For this review, take the finished solid that the model builds, in its own axes (mm). A direction names the side the tool comes from. Give positions to 0.01 mm unless a question says otherwise; leave off trailing zeros. Write each loop counter-clockwise with the first axis right and the second up, starting at its lowest first coordinate (ties: lowest second). Pieces come first, ordered by that corner, then holes. Notation, with made-up numbers: (-30, 22.5) -> (-4, 22.5) arc R22 ccw to (-4, 29.5) -> close; hole circle Ø11 at (83, 27). An arc over 180 degrees is marked (long way). Return JSON: item names as keys, results as strings.
from build123d import *

# Parameters (mm, degrees)
SKETCH1_W           = 139.457769838
SKETCH1_H           = 99.02864438
BOSS_EXTRUDE1_DEPTH = 10
BOSS_EXTRUDE2_DEPTH = 99.028644381
BOSS_EXTRUDE3_DEPTH = 99.028644381


with BuildPart() as part:
    # Sketch1 → Boss-Extrude1 (new body)
    with BuildSketch(Plane.XY):
        Rectangle(SKETCH1_W, SKETCH1_H)
    extrude(amount=BOSS_EXTRUDE1_DEPTH)

    # Sketch2 → Boss-Extrude2 (add)
    with BuildSketch(Plane(origin=(0, 49.51432219, 0), x_dir=(1, 0, 0), z_dir=(0, 1, 0))):
        Polygon((-69.728884919, 0), (41.491223437, 119.146703645), (25.829944634, 119.146703645), (-103.609221326, -10), (-69.728884919, -10), align=None)
    extrude(amount=-BOSS_EXTRUDE2_DEPTH)

    # Sketch3 → Boss-Extrude3 (add)
    with BuildSketch(Plane(origin=(0, 49.51432219, 0), x_dir=(1, 0, 0), z_dir=(0, 1, 0))):
        Polygon((41.491223437, 119.146703645), (41.491223437, 283.914864742), (-131.976237247, 283.914864742), (-131.976237247, 227.19452677), (25.829944634, 227.19452677), (25.829944634, 119.146703645), align=None)
    extrude(amount=-BOSS_EXTRUDE3_DEPTH)


solid = part.part
1. For pin 1 (2 mm diameter, centred on y = -25.5, z = -106, fed in from +X); pin 2 (8 mm diameter, centred on y = -5.5, z = -254.5, fed in from +X), all flat-tipped, find the tip position at first contact; note any pin that passes through.
Results found:
{"pin 1": "stops at x = 30.15", "pin 2": "stops at x = 41.49"}
2. The part is to be moulded in two halves that separate along Z. For faces 1 (the flat face through (25.83, 1, -174)), 2 (the flat face through (-44, 1, -283.915)), 3 (the flat face through (-47, 49.514, -236)), 4 (the flat face through (-1, 1, 0)), say which applies: +Z half, -Z half, draft (parallel to the pull), parting line (faces both ways), or undercut.
Results found:
{"face 1": "undercut", "face 2": "-Z half", "face 3": "draft", "face 4": "undercut"}
3. For faces 5 (the flat face through (-37.98, 0.69, -55.48)), 6 (the flat face through (41.491, 1, -200)), 7 (the flat face through (-14.897, 0.693, -58.739)), 8 (the flat face through (69.729, -1, 5)), list the 3-axis set-ups (+Z, -Z, +X, -X, +Y, -Y) from which the entire face can be reached by the end or side of a thin tool; tool diameter is ignored.
Results found:
{"face 5": "-X, +Y, -Y", "face 6": "-Z, +X, +Y, -Y", "face 7": "+X, +Y, -Y", "face 8": "+Z, -Z, +X, +Y, -Y"}
4. Add section B-B, the plane y = -17. State the section outline as (x, z) points.
Results found:
{"outline": "(-131.98, -283.91) -> (41.49, -283.91) -> (41.49, -119.15) -> (-69.73, 0) -> (69.73, 0) -> (69.73, 10) -> (-103.61, 10) -> (25.83, -119.15) -> (25.83, -227.19) -> (-131.98, -227.19) -> close"}
5. Add section A-A, the plane x = 33. State the section outline as (y, z) points.
Results found:
{"outline": "(-49.51, -283.91) -> (49.51, -283.91) -> (49.51, -110.05) -> (-49.51, -110.05) -> close; (-49.51, 0) -> (49.51, 0) -> (49.51, 10) -> (-49.51, 10) -> close"}
6. Add section C-C, the plane z = -238. State the section outline as (x, y) points, plus the area to 3 significant figures.
Results found:
{"outline": "(-131.98, -49.51) -> (41.49, -49.51) -> (41.49, 49.51) -> (-131.98, 49.51) -> close", "area": "17,200 mm²"}
7. To check wall thickness, follow probe 1 along Z at (x, y) = (12, -1.5); probe 2 along Z at (x, y) = (-27, 19.5); probe 3 along Z at (x, y) = (-120.5, 38). State the ranges of each line that lie inside material, in increasing order.
Results found:
{"probe 1": "z = -283.91 to -227.19, -105.35 to -87.55, 0 to 10", "probe 2": "z = -283.91 to -227.19, -66.44 to -45.77, 0 to 10", "probe 3": "z = -283.91 to -227.19"}
8. Add section D-D, the plane x = -110.5. State the section outline as (y, z) points.
Results found:
{"outline": "(-49.51, -283.91) -> (49.51, -283.91) -> (49.51, -227.19) -> (-49.51, -227.19) -> close"}
